The listing builds one solid part. Answer for the finished solid, in the listing's coordinates (mm). Face numbers are marked on the shaded views. A direction names the side the tool comes from. Give positions to 0.01 mm unless a question says otherwise; leave off trailing zeros. Loops run counter-clockwise (first coordinate to the right, second up) from the corner with the lowest first, then second, coordinate; pieces in that order, holes last. Notation, with made-up numbers: M 55,-3.75 L 71,-3.75 A22 ccw 71,10.25 Z; hole C 57.5,72.5 d1. An arc over 180 degrees is marked long. One line per item, written item: value. Start each with the question number.
Q1. A cutting plane is placed at B-B, the plane x = 25.75. Determine the outline of the cut face in (y, z), and give its area (3 significant figures).
Q2. A flat-ended cylindrical pin translates along its axis: pin 1 (1 mm diameter, centred on x = 20, z = 1, fed in from -Y). Find the tip coordinate at first contact, or state that the pin passes through.
Q3. Consider L1, parallel to Y at x = 27, z = 1.35; L2, parallel to Y at x = 33.75, z = 0.2; L3, parallel to X at y = 12.25, z = 2.6. Determine where each line is inside the solid, lowest interval first.
Q4. A cutting plane is placed at D-D, the plane y = 10.5. Determine the outline of the cut face in (x, z).
Q5. A cutting plane is placed at A-A, the plane y = 26.5. Determine the outline of the cut face in (x, z), and give its area (3 significant figures).
Q6. For the marked faces 4 and 5, determine the directions among +Z, -Z, +X, -X, +Y, -Y from which every point of the face is accessible in a straight line to the end or side of a thin tool.
Q7. A cutting plane is placed at C-C, the plane z = 1.2. Determine the outline of the cut face in (x, y), and give its area (3 significant figures).
Q8. The mould has two halves that part along Y. Classify the marked faces 1, 2 and 3: +Y half, -Y half, draft (parallel to the pull), parting line (faces both ways), or undercut.
from build123d import *

# Parameters (mm, degrees)
ESBO_O1_W                = 22.1
ESBO_O1_H                = 24.6
RESSALTO_EXTRUS_O1_DEPTH = 3
FILETE1_R                = 5


with BuildPart() as part:
    # Esboço1 → Ressalto-extrusão1 (new body)
    with BuildSketch(Plane.XY):
        with Locations((27.12188209, 20.25)):
            Rectangle(ESBO_O1_W, ESBO_O1_H)
        with BuildLine():
            Line((22.12188209, 28.55), (32.12188209, 28.55))
            ThreePointArc((32.12188209, 28.55), (34.17188209, 26.5), (32.12188209, 24.45))
            Line((32.12188209, 24.45), (22.12188209, 24.45))
            ThreePointArc((22.12188209, 24.45), (20.07188209, 26.5), (22.12188209, 28.55))
        make_face(mode=Mode.SUBTRACT)
        with BuildLine():
            Line((22.12188209, 16.05), (32.12188209, 16.05))
            ThreePointArc((32.12188209, 16.05), (34.17188209, 14), (32.12188209, 11.95))
            Line((32.12188209, 11.95), (22.12188209, 11.95))
            ThreePointArc((22.12188209, 11.95), (20.07188209, 14), (22.12188209, 16.05))
        make_face(mode=Mode.SUBTRACT)
    extrude(amount=RESSALTO_EXTRUS_O1_DEPTH)

    # Filete1
    filete1_edges = [part.edges().sort_by_distance(p)[0] for p in [
        (16.07188209, 32.55, 1.5),
        (38.17188209, 32.55, 1.5),
        (38.17188209, 7.95, 1.5),
        (16.07188209, 7.95, 1.5),
    ]]
    fillet(filete1_edges, radius=FILETE1_R)


solid = part.part
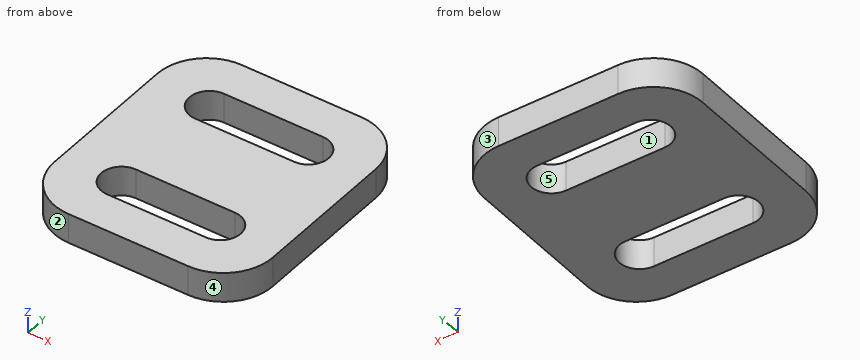
Answer block:
1. outline: M 7.95,0 L 11.95,0 L 11.95,3 L 7.95,3 Z; M 16.05,0 L 24.45,0 L 24.45,3 L 16.05,3 Z; M 28.55,0 L 32.55,0 L 32.55,3 L 28.55,3 Z
1. area: 49.2 mm^2
2. pin 1: y = 7.98
3. L1: 7.95 to 11.95, 16.05 to 24.45, 28.55 to 32.55
3. L2: 7.98 to 12.75, 15.25 to 25.25, 27.75 to 32.52
3. L3: 16.12 to 21.05, 33.19 to 38.12
4. outline: M 16.71,0 L 37.53,0 L 37.53,3 L 16.71,3 Z
5. outline: M 16.07,0 L 20.07,0 L 20.07,3 L 16.07,3 Z; M 34.17,0 L 38.17,0 L 38.17,3 L 34.17,3 Z
5. area: 24.0 mm^2
6. face 4: +Z, -Z, +X, -Y
6. face 5: +Z, -Z
7. outline: M 16.07,12.95 A5 ccw 21.07,7.95 L 33.17,7.95 A5 ccw 38.17,12.95 L 38.17,27.55 A5 ccw 33.17,32.55 L 21.07,32.55 A5 ccw 16.07,27.55 Z; hole M 22.12,11.95 L 32.12,11.95 A2.05 ccw 32.12,16.05 L 22.12,16.05 A2.05 ccw Z; hole M 22.12,24.45 L 32.12,24.45 A2.05 ccw 32.12,28.55 L 22.12,28.55 A2.05 ccw Z
7. area: 414 mm^2
8. face 1: undercut
8. face 2: -Y half
8. face 3: +Y half
